```python
from build123d import *

# Parameters (mm, degrees)
SKETCH5_W                = 33.357089
SKETCH5_H                = 38.1
BOSS_EXTRUDE2_DEPTH      = 20.8
BOSS_EXTRUDE2_DEPTH_BACK = 69.85
SKETCH6_W                = 84.3
SKETCH6_H                = 27.007089
CUT_EXTRUDE1_DEPTH       = 39.1
SKETCH7_R                = 3.5
CUT_EXTRUDE2_DEPTH       = 21.8
CUT_EXTRUDE2_DEPTH_BACK  = 70.85
CUT_EXTRUDE3_DEPTH       = 70.85
SKETCH9_W                = 28.5
SKETCH9_H                = 38.1
BOSS_EXTRUDE3_DEPTH      = 15
CUT_EXTRUDE4_DEPTH       = 70.85
SKETCH11_R               = 3.5
CUT_EXTRUDE5_DEPTH       = 70.85
SKETCH13_W               = 11.43
SKETCH13_H               = 25.4
CUT_EXTRUDE6_DEPTH       = 26.807089
CUT_EXTRUDE6_DEPTH_BACK  = 7.35


with BuildPart() as part:
    # Sketch5 → Boss-Extrude2 (new body, two sides)
    with BuildSketch(Plane(origin=(0, 0, 0), x_dir=(0, -1, 0), z_dir=(1, 0, 0))) as boss_extrude2_sk:
        with Locations((-10.3285445, 0)):
            Rectangle(SKETCH5_W, SKETCH5_H)
    extrude(amount=BOSS_EXTRUDE2_DEPTH)
    extrude(boss_extrude2_sk.sketch, amount=-BOSS_EXTRUDE2_DEPTH_BACK)

    # Sketch6 → Cut-Extrude1 (cut, through all)
    with BuildSketch(Plane.XY.offset(19.05)):
        with Locations((-21.35, 13.5035445)):
            Rectangle(SKETCH6_W, SKETCH6_H)
    extrude(amount=-CUT_EXTRUDE1_DEPTH, mode=Mode.SUBTRACT)

    # Sketch7 → Cut-Extrude2 (cut, two sides)
    with BuildSketch(Plane(origin=(0, 0, 0), x_dir=(0, 0, -1), z_dir=(1, 0, 0))) as cut_extrude2_sk:
        with Locations((0, 14.307089)):
            Circle(SKETCH7_R)
    extrude(amount=CUT_EXTRUDE2_DEPTH, mode=Mode.SUBTRACT)
    extrude(cut_extrude2_sk.sketch, amount=-CUT_EXTRUDE2_DEPTH_BACK, mode=Mode.SUBTRACT)

    # Sketch8 → Cut-Extrude3 (cut, through all)
    with BuildSketch(Plane(origin=(0, 0, 0), x_dir=(0, 0, -1), z_dir=(1, 0, 0))):
        with BuildLine():
            Line((19.05, 0), (10.486875479, 19.026775715))
            ThreePointArc((10.486875479, 19.026775715), (0, 25.807089), (-10.486875479, 19.026775715))
            Line((-10.486875479, 19.026775715), (-19.05, 0))
            Line((-19.05, 0), (-19.05, 27.007089))
            Line((-19.05, 27.007089), (19.05, 27.007089))
            Line((19.05, 27.007089), (19.05, 0))
        make_face()
    extrude(amount=-CUT_EXTRUDE3_DEPTH, mode=Mode.SUBTRACT)

    # Sketch9 → Boss-Extrude3 (add)
    with BuildSketch(Plane(origin=(0, 0, 0), x_dir=(1, 0, 0), z_dir=(0, 1, 0))):
        with Locations((-49.25, 0)):
            Rectangle(SKETCH9_W, SKETCH9_H)
    extrude(amount=BOSS_EXTRUDE3_DEPTH)

    # Sketch10 → Cut-Extrude4 (cut, through all)
    with BuildSketch(Plane(origin=(0, 0, 0), x_dir=(0, 0, -1), z_dir=(1, 0, 0))):
        Polygon((19.05, 42.328016658), (19.05, 0), (0, 42.328016658), align=None)
        Polygon((-19.05, 42.328016658), (0, 42.328016658), (-19.05, 0), align=None)
    extrude(amount=-CUT_EXTRUDE4_DEPTH, mode=Mode.SUBTRACT)

    # Sketch11 → Cut-Extrude5 (cut, through all)
    with BuildSketch(Plane(origin=(0, 0, 0), x_dir=(0, 0, -1), z_dir=(1, 0, 0))):
        with Locations((0, 14.307089)):
            Circle(SKETCH11_R)
    extrude(amount=-CUT_EXTRUDE5_DEPTH, mode=Mode.SUBTRACT)

    # Sketch13 → Cut-Extrude6 (cut, two sides)
    with BuildSketch(Plane(origin=(0, 0, 0), x_dir=(1, 0, 0), z_dir=(0, 1, 0))) as cut_extrude6_sk:
        with Locations((-46.715, -19.05)):
            Rectangle(SKETCH13_W, SKETCH13_H)
        with Locations((-46.715, 19.05)):
            Rectangle(SKETCH13_W, SKETCH13_H)
    extrude(amount=CUT_EXTRUDE6_DEPTH, mode=Mode.SUBTRACT)
    extrude(cut_extrude6_sk.sketch, amount=-CUT_EXTRUDE6_DEPTH_BACK, mode=Mode.SUBTRACT)


solid = part.part
```
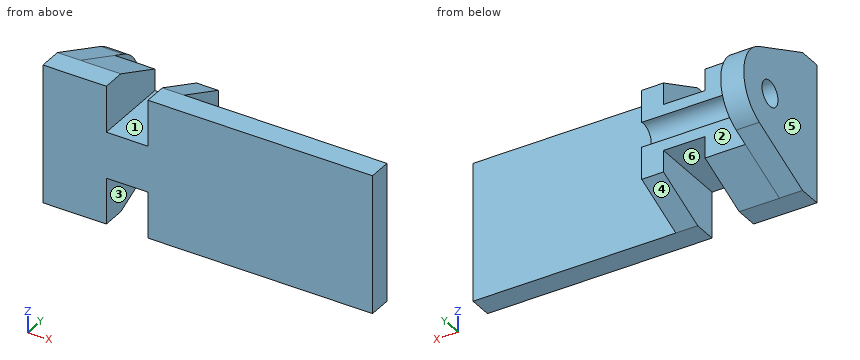
Work out the finished part from the listing and answer in its coordinate system (mm). Face numbers are marked on the shaded views. A direction names the side the tool comes from. Round coordinates to 2 decimals unless told otherwise and drop trailing zeros. Write each loop counter-clockwise with the first axis right and the second up, starting at its lowest first coordinate (ties: lowest second). Pieces come first, ordered by that corner, then holes. Notation, with made-up numbers: (3.25, 19.25) - (62.25, 19.25) arc R11 cw to (62.25, 24.25) - close; hole circle Ø4 at (27, 78.5). An arc over 180 degrees is marked (long way). Return JSON: item names as keys, results as strings. Group by question number.
Q1. For the marked faces 1, 2 and 3, determine the directions among +Z, -Z, +X, -X, +Y, -Y from which every point of the face is accessible in a straight line to the end or side of a thin tool.
Q2. The part is cut by section C-C on y = 16.5. Write down the section's boundary in (x, z).
Q3. The part is cut by section B-B on y = -3. Write down the section's boundary in (x, z).
Q4. The part is cut by section A-A on z = 0. Write down the section's boundary in (x, y), then the cut area to 3 significant figures.
Q5. The mould has two halves that part along X. Classify the marked faces 4, 5 and 6: released by +X, released by -X, zero draft, split by the parting line, or undercut.
Q6. Find the intervals of material crossed by L1, parallel to X at y = 7.5, z = 8.5; L2, parallel to X at y = -4, z = -16; L3, parallel to Y at x = -54.5, z = 0, in increasing order.
Q7. Each of these flat-tipped pins is pushed along its axis until it touches: pin 1 Ø3 at (y, z) = (19, 5) entering from +X; pin 2 Ø3 at (x, y) = (-58, 8) entering from +Z; pin 3 Ø12 at (y, z) = (12.5, 12.5) entering from +X. Where does it stop, or does it pass through?
Q8. The part is cut by section D-D on z = -17. Write down the section's boundary in (x, y), then the cut area to 3 significant figures.
Solved:
{
 "1": {"face 1": "+Z, +Y, -Y", "face 2": "+Z, -Z, +X, +Y", "face 3": "-Z, +Y, -Y"},
 "2": {"outline": "(-69.85, -11.62) - (-63.5, -11.62) - (-63.5, -2.73) - (-69.85, -2.73) - close; (-69.85, 2.73) - (-63.5, 2.73) - (-63.5, 11.62) - (-69.85, 11.62) - close"},
 "3": {"outline": "(-69.85, -19.05) - (-52.43, -19.05) - (-52.43, -6.35) - (-41, -6.35) - (-41, -19.05) - (20.8, -19.05) - (20.8, 19.05) - (-41, 19.05) - (-41, 6.35) - (-52.43, 6.35) - (-52.43, 19.05) - (-69.85, 19.05) - close"},
 "4": {"outline": "(-69.85, -6.35) - (20.8, -6.35) - (20.8, 0) - (-35, 0) - (-35, 10.81) - (-69.85, 10.81) - close; (-69.85, 17.81) - (-63.5, 17.81) - (-63.5, 25.81) - (-69.85, 25.81) - close", "area": "1,000 mm²"},
 "5": {"face 4": "zero draft", "face 5": "released by -X", "face 6": "undercut"},
 "6": {"L1": "-69.85 to -52.43, -41 to -35", "L2": "-69.85 to -52.43, -41 to 20.8", "L3": "-6.35 to 10.81"},
 "7": {"pin 1": "x = -63.5", "pin 2": "z = 16.12", "pin 3": "x = -35"},
 "8": {"outline": "(-69.85, -6.35) - (-52.43, -6.35) - (-52.43, 4.55) - (-69.85, 4.55) - close; (-41, -6.35) - (20.8, -6.35) - (20.8, 0) - (-35, 0) - (-35, 4.55) - (-41, 4.55) - close", "area": "610 mm²"}
}
